Design review of the part built by this model. Coordinates are the model's own, in mm. Face numbers are marked on the shaded views. A direction names the side the tool comes from. Give positions to 0.01 mm unless a question says otherwise; leave off trailing zeros. One line per item, written item: value.
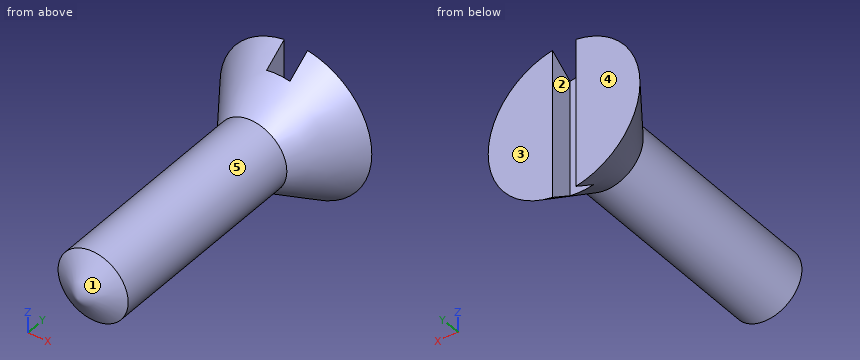
from build123d import *

# Parameters (mm, degrees)
SKETCH4_W               = 2
SKETCH4_H               = 3
CUT_EXTRUDE1_DEPTH      = 7.5
CUT_EXTRUDE1_DEPTH_BACK = 7.5


with BuildPart() as part:
    # Sketch3 → Revolve1 (revolve)
    with BuildSketch(Plane.XY):
        Polygon((0, 0), (3, 1.732050808), (3, 19.732050808), (6.5, 24.732050808), (0, 24.732050808), align=None)
    revolve(axis=Axis((0, -8.000817712, 0), (0, 1, 0)))

    # Sketch4 → Cut-Extrude1 (cut, two sides)
    with BuildSketch(Plane.XY) as cut_extrude1_sk:
        with Locations((0, 24.232050808)):
            Rectangle(SKETCH4_W, SKETCH4_H)
    extrude(amount=CUT_EXTRUDE1_DEPTH, mode=Mode.SUBTRACT)
    extrude(cut_extrude1_sk.sketch, amount=-CUT_EXTRUDE1_DEPTH_BACK, mode=Mode.SUBTRACT)


solid = part.part
Item 1: Clearance check with flat-ended pins moving along their axes: P1, Ø2, axis at x = 1.5, y = 5, coming from the -Z side; P2, Ø1, axis at y = 23.5, z = 1.5, coming from the +X side; P3, Ø2, axis at y = 23, z = -1.5, coming from the -X side. State where each tip first meets the part, or that it passes through.
Returned:
P1: z = -2.96
P2: x = 5.82
P3: x = -5.83
Item 2: Draft analysis for pull direction X (two halves, no side actions). For the marked faces 1, 2 and 3, state which applies: pulls with the +X half, pulls with the -X half, needs draft (parallel to the pull), parting line crosses it, or undercut.
Returned:
face 1: parting line crosses it
face 2: undercut
face 3: needs draft
Item 3: Machinability: for the marked faces 4 and 5, which of the approach directions +Z, -Z, +X, -X, +Y, -Y give a long, thin tool a straight path to every point of the face, cutting with its end or side? Answer none if there is none.
Returned:
face 4: +Z, -Z, +X, -X, +Y
face 5: -Y
Item 4: To check wall thickness, follow line 1 along Z through (x, y) = (1, 10); line 2 along X through (y, z) = (21, -1.75); line 3 along Y through (x, z) = (2.75, -1.5). State the ranges of each line that lie inside material, in increasing order. Write a range as from..to.
Returned:
line 1: -2.83..2.83
line 2: -3.47..3.47
line 3: 19.92..24.73
